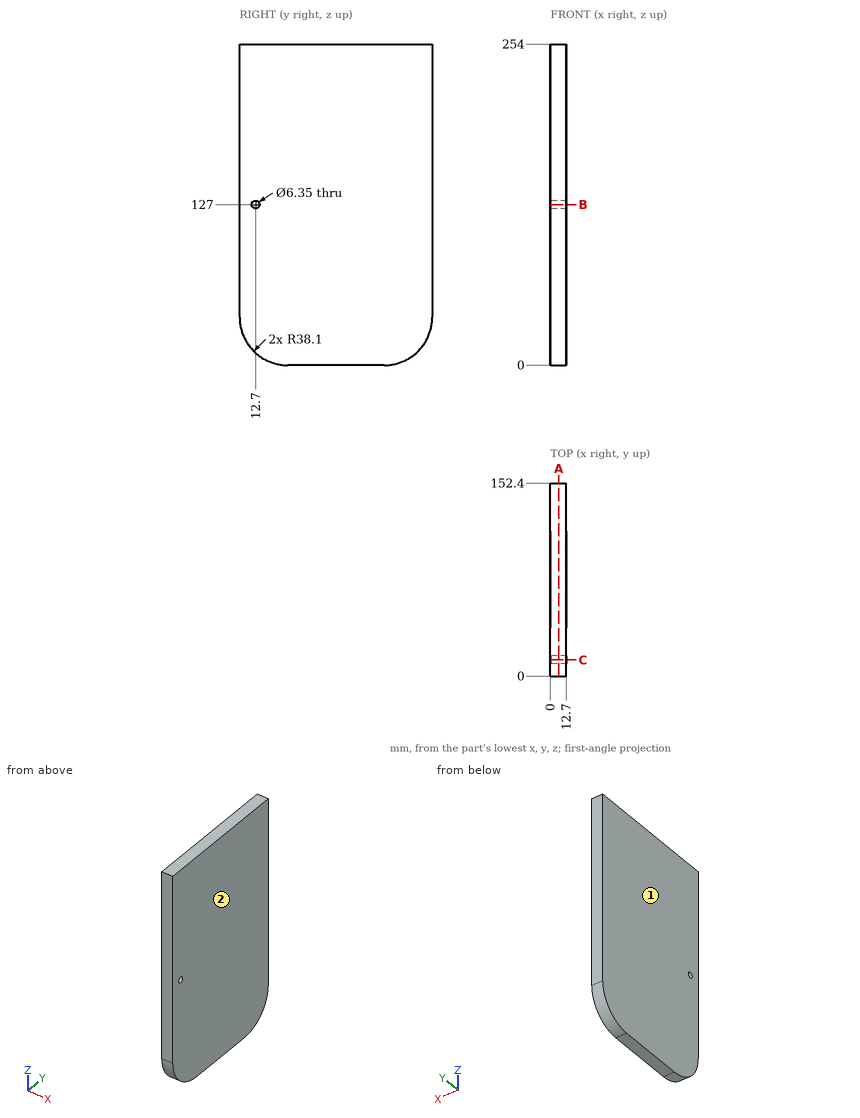
Design review of the part shown in the three views and the two pictorial views. Dimensions are in mm from the part's minimum x, y and z. Round coordinates to 2 decimals unless told otherwise and drop trailing zeros. Write each loop counter-clockwise with the first axis right and the second up, starting at its lowest first coordinate (ties: lowest second). Pieces come first, ordered by that corner, then holes. Notation, with made-up numbers: (-39, 78.5) -> (1, 78.5) arc R36 ccw to (1, 114.5) -> close; hole circle Ø2 at (56.5, 57.5). An arc over 180 degrees is marked (long way). One line per question, with ' | ' between items. Start each with the question number.
1) Mouldability with a two-part tool opening along X and no side actions: class the marked faces 1 and 2 as +X half, -X half, draft (parallel to the pull), parting line (faces both ways), or undercut.
2) Wall thickness on line 1 along Y through (x, z) = (5, 127) (3 decimals); line 2 along Z through (x, y) = (9.5, 12.7) (3 decimals); line 3 along Z through (x, y) = (4, 30.5): over which ranges is each line inside the solid? List them lowest first.
3) For pin 1 Ø1 at (x, y) = (10, 130) entering from -Z; pin 2 Ø1 at (x, y) = (2.5, 120) entering from -Z; pin 3 Ø1 at (x, y) = (9, 116.5) entering from -Z, all flat-tipped, find the tip position at first contact; note any pin that passes through.
4) Add section C-C (y = 12.7). Write out the cut boundary in (x, z) (3 decimals), and give its area (3 significant figures).
5) Add section A-A (x = 6.75). Write out the cut boundary in (y, z) (3 decimals), and give its area (3 significant figures).
6) Add section B-B (z = 127). Write out the cut boundary in (x, y) (3 decimals).
Reported:
1) face 1: -X half | face 2: +X half
2) line 1: y = 0 to 9.525, 15.875 to 152.4 | line 2: z = 9.702 to 123.825, 130.175 to 254 | line 3: z = 0.77 to 254
3) pin 1: stops at z = 3.16 | pin 2: stops at z = 0.36 | pin 3: stops at z = 0.04
4) outline: (0, 9.702) -> (12.7, 9.702) -> (12.7, 123.825) -> (0, 123.825) -> close; (0, 130.175) -> (12.7, 130.175) -> (12.7, 254) -> (0, 254) -> close | area: 3,020 mm²
5) outline: (0, 38.1) arc R38.1 ccw to (38.1, 0) -> (114.3, 0) arc R38.1 ccw to (152.4, 38.1) -> (152.4, 254) -> (0, 254) -> close; hole circle Ø6.35 at (12.7, 127) | area: 38,100 mm²
6) outline: (0, 0) -> (12.7, 0) -> (12.7, 9.525) -> (0, 9.525) -> close; (0, 15.875) -> (12.7, 15.875) -> (12.7, 152.4) -> (0, 152.4) -> close
